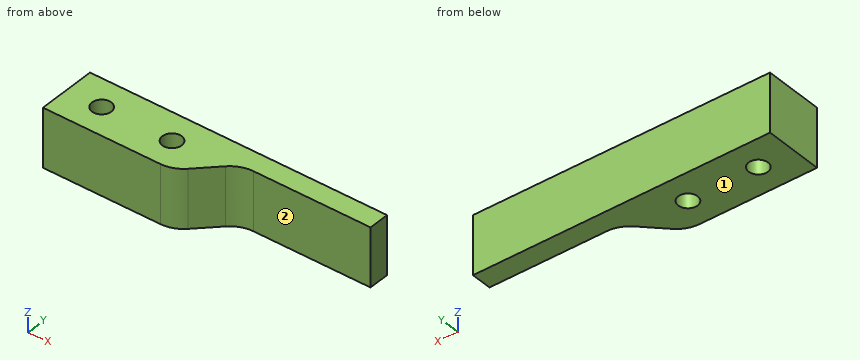
from build123d import *

# Parameters (mm, degrees)
EXTRUDE_1_DEPTH    = 10
HOLE_WIZARD_M4_1_D = 3.3


with BuildPart() as part:
    # 草图5 → 凸台-拉伸1 (new body)
    with BuildSketch(Plane.XY):
        with BuildLine():
            Line((7834.715889536, 44.670845652), (7854.715889536, 44.670845652))
            ThreePointArc((7854.715889536, 44.670845652), (7856.629306698, 45.05144799), (7858.251423442, 46.135311746))
            Line((7858.251423442, 46.135311746), (7861.822491254, 49.706379558))
            ThreePointArc((7861.822491254, 49.706379558), (7863.444607998, 50.790243315), (7865.358025159, 51.170845652))
            Line((7865.358025159, 51.170845652), (7885.358025159, 51.170845652))
            Line((7885.358025159, 51.170845652), (7885.358025159, 54.670845652))
            Line((7885.358025159, 54.670845652), (7834.715889536, 54.670845652))
            Line((7834.715889536, 54.670845652), (7834.715889536, 44.670845652))
        make_face()
    extrude(amount=EXTRUDE_1_DEPTH)

    # M4 螺纹孔1 (through all)
    with Locations(Plane.XY.offset(10)):
        with Locations((7840.715889536, 49.670845652), (7852.715889536, 49.670845652)):
            Hole(HOLE_WIZARD_M4_1_D / 2)


solid = part.part
Read the model definition and answer for the solid it produces. Units are mm, in the model's axes. Face numbers are marked on the shaded views. A direction names the side the tool comes from. Round coordinates to 2 decimals unless told otherwise and drop trailing zeros. Write each loop counter-clockwise with the first axis right and the second up, starting at its lowest first coordinate (ties: lowest second). Pieces come first, ordered by that corner, then holes. Notation, with made-up numbers: (57.5, 61) - (106.5, 61) arc R22 cw to (106.5, 100) - close; hole circle Ø8 at (34.25, -16). An arc over 180 degrees is marked (long way). Use a Markdown table: item, result.
(1) The part is cut by section B-B (z = 7.5). Write down the section's boundary in (x, y), then the cut area to 3 significant figures.
Reported:
| item | result |
|---|---|
| outline | (7834.72, 44.67) - (7854.72, 44.67) arc R5 ccw to (7858.25, 46.14) - (7861.82, 49.71) arc R5 cw to (7865.36, 51.17) - (7885.36, 51.17) - (7885.36, 54.67) - (7834.72, 54.67) - close; hole circle Ø3.3 at (7840.72, 49.67); hole circle Ø3.3 at (7852.72, 49.67) |
| area | 325 mm2 |
(2) Which of the six approach directions +Z, -Z, +X, -X, +Y, -Y give full straight-line access (tool end or side, diameter ignored) to the marked faces 1 and 2?
Reported:
| item | result |
|---|---|
| face 1 | -Z, +X, -X, +Y, -Y |
| face 2 | +Z, -Z, +X, -Y |
(3) The part is cut by section A-A (x = 7853.5). Write down the section's boundary in (y, z), then the cut area to 3 significant figures.
Reported:
| item | result |
|---|---|
| outline | (44.67, 0) - (48.22, 0) - (48.22, 10) - (44.67, 10) - close; (51.12, 0) - (54.67, 0) - (54.67, 10) - (51.12, 10) - close |
| area | 71.0 mm2 |
(4) The part is cut by section C-C (x = 7869). Write down the section's boundary in (y, z), then the cut area to 3 significant figures.
Reported:
| item | result |
|---|---|
| outline | (51.17, 0) - (54.67, 0) - (54.67, 10) - (51.17, 10) - close |
| area | 35.0 mm2 |
(5) Each of these flat-tipped pins is pushed along its axis until it touches: pin 1 Ø3 at (x, z) = (7877.5, 3.5) entering from -Y; pin 2 Ø6 at (x, y) = (7879.5, 47) entering from +Z. Where does it stop, or does it pass through?
Reported:
| item | result |
|---|---|
| pin 1 | y = 51.17 |
| pin 2 | through |
(6) The part is cut by section D-D (y = 47). Write down the section's boundary in (x, z).
Reported:
| item | result |
|---|---|
| outline | (7834.72, 0) - (7859.12, 0) - (7859.12, 10) - (7834.72, 10) - close |
(7) Straight lines are drawn through the part: line 1 along X through (y, z) = (50.5, 8); line 2 along Y through (x, z) = (7880.5, 7.5); line 3 along Y through (x, z) = (7855, 6.75). For each, find the intervals that lie inside material, in ascending order. Write a range as [from, to].
Reported:
| item | result |
|---|---|
| line 1 | [7834.72, 7839.29], [7842.14, 7851.29], [7854.14, 7862.86] |
| line 2 | [51.17, 54.67] |
| line 3 | [44.68, 54.67] |
